```python
from build123d import *

# Parameters (mm, degrees)
EXTRUIR1_DEPTH = 10
CROQUIS5_W     = 4
CROQUIS5_H     = 2.45
EXTRUIR2_DEPTH = 4
REDONDEO1_R    = 2
CROQUIS6_R     = 1
EXTRUIR3_DEPTH = 4


with BuildPart() as part:
    # Croquis4 → Extruir1 (new body)
    with BuildSketch(Plane.XY):
        Polygon((32.33206977, 6.125), (31.10367023, 9.5), (30.157386445, 9.5), (28.928986905, 6.125), (27.619680795, 6.125), (26.391281255, 9.5), (25.44499747, 9.5), (24.21659793, 6.125), (22.90729182, 6.125), (21.67889228, 9.5), (20.732608495, 9.5), (19.504208955, 6.125), (18.194902845, 6.125), (16.966503305, 9.5), (16.02021952, 9.5), (14.79181998, 6.125), (13.48251387, 6.125), (12.25411433, 9.5), (11.307830545, 9.5), (10.079431005, 6.125), (8.770124895, 6.125), (7.541725355, 9.5), (6.59544157, 9.5), (5.36704203, 6.125), (4.05773592, 6.125), (2.82933638, 9.5), (1.883052595, 9.5), (0.654653055, 6.125), (0, 6.125), (0, 0), (37.6991118, 0), (37.6991118, 6.125), (37.044458745, 6.125), (35.816059205, 9.5), (34.86977542, 9.5), (33.64137588, 6.125), align=None)
    extrude(amount=EXTRUIR1_DEPTH)

    # Croquis5 → Extruir2 (add)
    with BuildSketch(Plane(origin=(37.6991118, 0, 0), x_dir=(0, 0, -1), z_dir=(1, 0, 0))):
        with Locations((-5, 3.0625)):
            Rectangle(CROQUIS5_W, CROQUIS5_H)
    extruir2 = extrude(amount=EXTRUIR2_DEPTH)

    # Simetría1: Extruir2 across plane
    add(extruir2.mirror(Plane(origin=(18.8495559, 0, 0), x_dir=(0, 0, 1), z_dir=(1, 0, 0))))

    # Redondeo1
    redondeo1_edges = [part.edges().sort_by_distance(p)[0] for p in [
        (41.6991118, 3.0625, 7),
        (41.6991118, 3.0625, 3),
        (-4, 3.0625, 3),
        (-4, 3.0625, 7),
    ]]
    fillet(redondeo1_edges, radius=REDONDEO1_R - 0.0001)  # a hair under: the kernel refuses the full size

    # Croquis6 → Extruir3 (cut)
    with BuildSketch(Plane(origin=(0, 4.2875, 0), x_dir=(1, 0, 0), z_dir=(0, 1, 0))):
        with Locations(Location((39.6991118, -5, 0), (0, 0, 270))):
            Circle(CROQUIS6_R)
        with Locations(Location((-2, -5, 0), (0, 0, 270))):
            Circle(CROQUIS6_R)
    extrude(amount=-EXTRUIR3_DEPTH, mode=Mode.SUBTRACT)


solid = part.part
```
Geometry check sheet. Reference: the model listing, model coordinates, mm. A direction names the side the tool comes from. Round coordinates to 2 decimals unless told otherwise and drop trailing zeros. Write each loop counter-clockwise with the first axis right and the second up, starting at its lowest first coordinate (ties: lowest second). Pieces come first, ordered by that corner, then holes. Notation, with made-up numbers: (55.25, 3.5) -> (106.25, 3.5) arc R34 ccw to (106.25, 41.5) -> close; hole circle Ø3 at (3.5, 68). An arc over 180 degrees is marked (long way). Put each result on its own line as item: value.
1) Cross-section at A-A, the plane y = 6.75. Give the number of separate pieces and of enclosed holes in the cut face, plus the area to 3 significant figures.
Recorded:
separate pieces: 8
enclosed holes: 0
area: 236 mm2
2) Depth check by flat-ended pin: P1, Ø1.2, axis at x = -3, z = 4.5, coming from the -Y side; P2, Ø1.5, axis at y = 3, z = 8, coming from the -X side; P3, Ø1.8, axis at y = 2, z = 3, coming from the +X side. Enter the tip coordinate at first touch or a pass-through.
Recorded:
P1: stops at y = 1.84
P2: stops at x = 0
P3: stops at x = 41.37
3) Cross-section at C-C, the plane x = 8. Enter the section's corners in (y, z).
Recorded:
outline: (0, 0) -> (8.24, 0) -> (8.24, 10) -> (0, 10) -> close
4) Thickness scan on probe 1 along X at (y, z) = (2.85, 5); probe 2 along Y at (x, z) = (0.5, 3.25) (3 decimals); probe 3 along X at (y, z) = (3, 4.5). Record the ranges inside material, lowest first. Write a range as from..to.
Recorded:
probe 1: x = -4..-3, -1..38.7, 40.7..41.7
probe 2: y = 0..6.125
probe 3: x = -3.94..-2.87, -1.13..38.83, 40.57..41.64
5) Access from +Z, -Z, +X, -X, +Y, -Y to the whole of each face (thin tool, end or side, straight path). Record for faces 1 (the face through (36.44, 7.79, 4.93)), 2 (the face through (17.59, 7.79, 4.93)), 3 (the face through (-1, 3, 3)), 4 (the face through (39, 3, 7)), 5 (the face through (1.28, 7.84, 4.93)).
Recorded:
face 1: +Z, -Z, +X, +Y
face 2: +Z, -Z, +Y
face 3: -Z, -X, +Y, -Y
face 4: +Z, +X, +Y, -Y
face 5: +Z, -Z, -X, +Y
